```python
from build123d import *

# Parameters (mm, degrees)
EXTRUDE_1_DEPTH      = 7
SKETCH_4_W           = 12.5
SKETCH_4_H           = 12.5
CUT_EXTRUDE_1_DEPTH  = 5.5
SKETCH_5_R           = 2.6
SKETCH_5_R_2         = 6.5
CUT_EXTRUDE_2_DEPTH  = 64.474798149
SKETCH_6_R           = 1
CUT_EXTRUDE_3_DEPTH  = 64.474798149
EXTRUDE_2_DEPTH      = 7
SKETCH_9_W           = 12
SKETCH_9_H           = 12
CUT_EXTRUDE_5_DEPTH  = 5
SKETCH_10_R          = 2.75
CUT_EXTRUDE_6_DEPTH  = 16
SKETCH_11_W          = 6.086395164
SKETCH_11_H          = 5.94224859
CUT_EXTRUDE_7_DEPTH  = 10
SKETCH_13_W          = 6.086395164
SKETCH_13_H          = 2.190675797
CUT_EXTRUDE_8_DEPTH  = 10
SKETCH_14_R          = 1.5
CUT_EXTRUDE_9_DEPTH  = 10
FILLET_1_R           = 0.3
FILLET_2_R           = 0.3
SKETCH_15_R          = 5
SKETCH_15_R_2        = 8.5
CUT_EXTRUDE_10_DEPTH = 1


with BuildPart() as part:
    # Эскиз1 → Бобышка-Вытянуть1 (new body)
    with BuildSketch(Plane.XY):
        with BuildLine():
            Line((0, 0), (50, 0))
            ThreePointArc((50, 0), (59.9, -9.9), (50, -19.8))
            Line((50, -19.8), (0, -19.8))
            ThreePointArc((0, -19.8), (-9.9, -9.9), (0, 0))
        make_face()
    extrude(amount=EXTRUDE_1_DEPTH)

    # Эскиз4 → Вырез-Вытянуть1 (cut)
    with BuildSketch(Plane.XY.offset(7)):
        with Locations((13.25, -9.9)):
            Rectangle(SKETCH_4_W, SKETCH_4_H)
        with Locations((28.75, -9.9)):
            Rectangle(SKETCH_4_W, SKETCH_4_H)
    extrude(amount=-CUT_EXTRUDE_1_DEPTH, mode=Mode.SUBTRACT)

    # Эскиз5 → Вырез-Вытянуть2 (cut, through all)
    with BuildSketch(Plane.XY.offset(7)):
        with Locations((0, -9.9)):
            Circle(SKETCH_5_R)
        with Locations((50, -9.9)):
            Circle(SKETCH_5_R_2)
    extrude(amount=-CUT_EXTRUDE_2_DEPTH, mode=Mode.SUBTRACT)

    # Эскиз6 → Вырез-Вытянуть3 (cut, through all)
    with BuildSketch(Plane.XY.offset(7)):
        with Locations((10.5, -3.65)):
            Circle(SKETCH_6_R)
        with Locations((15.5, -3.65)):
            Circle(SKETCH_6_R)
        with Locations((26, -3.65)):
            Circle(SKETCH_6_R)
        with Locations((31, -3.65)):
            Circle(SKETCH_6_R)
        with Locations((10.5, -16.15)):
            Circle(SKETCH_6_R)
        with Locations((15.5, -16.15)):
            Circle(SKETCH_6_R)
        with Locations((26, -16.15)):
            Circle(SKETCH_6_R)
        with Locations((31, -16.15)):
            Circle(SKETCH_6_R)
    extrude(amount=-CUT_EXTRUDE_3_DEPTH, mode=Mode.SUBTRACT)

    # Эскиз8 → Бобышка-Вытянуть2 (add)
    with BuildSketch(Plane.XY.offset(7)):
        with BuildLine():
            Line((0, 2.1), (50, 2.1))
            ThreePointArc((50, 2.1), (62, -9.9), (50, -21.9))
            Line((50, -21.9), (0, -21.9))
            ThreePointArc((0, -21.9), (-12, -9.9), (0, 2.1))
        make_face()
        with BuildLine():
            Line((0, -0.209438441), (50, -0.209438441))
            ThreePointArc((50, -0.209438441), (59.690561559, -9.9), (50, -19.590561559))
            Line((50, -19.590561559), (0, -19.590561559))
            ThreePointArc((0, -19.590561559), (-9.690561559, -9.9), (0, -0.209438441))
        make_face(mode=Mode.SUBTRACT)
    extrude(amount=-EXTRUDE_2_DEPTH)

    # Эскиз9 → Вырез-Вытянуть5 (cut)
    with BuildSketch(Plane(origin=(0, 0, 0), x_dir=(-1, 0, 0), z_dir=(0, 0, -1))):
        with Locations((0, -9.9)):
            Rectangle(SKETCH_9_W, SKETCH_9_H)
    extrude(amount=-CUT_EXTRUDE_5_DEPTH, mode=Mode.SUBTRACT)

    # Эскиз10 → Вырез-Вытянуть6 (cut)
    with BuildSketch(Plane.XZ.offset(21.9)):
        with Locations((39, 4.7)):
            Circle(SKETCH_10_R)
    extrude(amount=-CUT_EXTRUDE_6_DEPTH, mode=Mode.SUBTRACT)

    # Эскиз11 → Вырез-Вытянуть7 (cut)
    with BuildSketch(Plane.XZ.offset(21.9)):
        with Locations((39, 4.7)):
            Rectangle(SKETCH_11_W, SKETCH_11_H)
    extrude(amount=-CUT_EXTRUDE_7_DEPTH, mode=Mode.SUBTRACT)

    # Эскиз13 → Вырез-Вытянуть8 (cut)
    with BuildSketch(Plane.XY.offset(1.728875705)):
        with Locations((39, -20.804662101)):
            Rectangle(SKETCH_13_W, SKETCH_13_H)
    extrude(amount=-CUT_EXTRUDE_8_DEPTH, mode=Mode.SUBTRACT)

    # Эскиз14 → Вырез-Вытянуть9 (cut)
    with BuildSketch(Plane.XY.offset(7)):
        with Locations((21, -1.9)):
            Circle(SKETCH_14_R)
        with Locations((21, -17.9)):
            Circle(SKETCH_14_R)
        with Locations((43, -1.9)):
            Circle(SKETCH_14_R)
        with Locations((-7, -9.9857634)):
            Circle(SKETCH_14_R)
        with Locations((43, -17.9)):
            Circle(SKETCH_14_R)
    extrude(amount=-CUT_EXTRUDE_9_DEPTH, mode=Mode.SUBTRACT)

    # Скругление1
    fillet_1_edges = [part.edges().sort_by_distance(p)[0] for p in [
        (-6, -8.867729411, 2.5),
        (-6, -11.103797388, 2.5),
    ]]
    fillet(fillet_1_edges, radius=FILLET_1_R)

    # Скругление2
    fillet_2_edges = [part.edges().sort_by_distance(p)[0] for p in [
        (42.043197582, -16.744781781, 4.364437853),
        (42.043197582, -19.055218219, 4.364437853),
    ]]
    fillet(fillet_2_edges, radius=FILLET_2_R)

    # Эскиз15 → Вырез-Вытянуть10 (cut)
    with BuildSketch(Plane.XY.offset(7)):
        with Locations((0, -9.9)):
            Circle(SKETCH_15_R)
        with Locations((50, -9.9)):
            Circle(SKETCH_15_R_2)
    extrude(amount=-CUT_EXTRUDE_10_DEPTH, mode=Mode.SUBTRACT)


solid = part.part
```
Read the model definition and answer for the solid it produces. Units are mm, in the model's axes. A direction names the side the tool comes from. Coordinates: 2 decimals unless noted, no trailing zeros. Order: outer loops, then holes, each group sorted by start corner. A loop starts at its lowest first (then second) coordinate and runs counter-clockwise, first axis right, second up. Notation, with made-up numbers: (83, 17.25) - (131, 17.25) arc R11 ccw to (131, 37.25) - close; hole circle Ø2 at (-5, -11). An arc over 180 degrees is marked (long way). Answer as a JSON object with one key per item and string values. Group by question number.
Item 1: Section A-A (x = 15.5) is taken. Give the vertices of the cut face in (y, z).
Item 2: Section B-B (x = 29) is taken. Give the vertices of the cut face in (y, z).
Item 3: Section D-D (z = 3) is taken. State how many separate pieces and enclosed holes the cut face has, plus the area to 3 significant figures.
Item 4: A tool of negligible diameter and unlimited length cuts with its end or side. For faces 3 (the face through (0, -3.9, 2)), 4 (the face through (24, -16.15, 4)), 5 (the face through (39, -19.709, 1)), from which of +Z, -Z, +X, -X, +Y, -Y can it reach the whole face along a straight path? Write none if from no direction.
Item 5: Consider probe 1 along X at (y, z) = (-9.75, 1); probe 2 along Y at (x, z) = (31, 3.25); probe 3 along X at (y, z) = (-2, 3.25). Determine where each line is inside the solid, lowest interval first. Write a range as from..to.
Item 6: The mould has two halves that part along Z. Classify faces 1 (the face through (2, -12, 6)), 2 (the face through (33, -16.15, 4)): +Z half, -Z half, draft (parallel to the pull), parting line (faces both ways), or undercut.
Item 7: Flat-ended cylindrical pins translate along their axes: P1, Ø3.5, axis at y = -13, z = 3, coming from the +X side; P2, Ø3, axis at y = -4, z = 1, coming from the +X side; P3, Ø0.9, axis at x = 40, z = 1, coming from the -Y side; P4, Ø1.8, axis at x = 15.5, y = -16.15, coming from the +Z side. Find the tip coordinate at first contact, or state that the pin passes through.
Item 8: Section C-C (x = 51) is taken. Give the vertices of the cut face in (y, z).
Results are:
{
 "1": {"outline": "(-21.9, 0) - (-17.15, 0) - (-17.15, 7) - (-21.9, 7) - close; (-15.15, 0) - (-4.65, 0) - (-4.65, 1.5) - (-15.15, 1.5) - close; (-2.65, 0) - (2.1, 0) - (2.1, 7) - (-2.65, 7) - close"},
 "2": {"outline": "(-21.9, 0) - (2.1, 0) - (2.1, 7) - (-3.65, 7) - (-3.65, 1.5) - (-16.15, 1.5) - (-16.15, 7) - (-21.9, 7) - close"},
 "3": {"separate pieces": "1", "enclosed holes": "7", "area": "930 mm^2"},
 "4": {"face 3": "-Z", "face 4": "+Z", "face 5": "+Z, -Z, -Y"},
 "5": {"probe 1": "x = -12..-8.48, 6..43.5, 56.5..62", "probe 2": "y = -21.9..-17.15, -2.65..2.1", "probe 3": "x = -9.03..19.5, 22.5..41.5, 44.5..59.03"},
 "6": {"face 1": "+Z half", "face 2": "draft"},
 "7": {"P1": "stops at x = 61.92", "P2": "stops at x = 61.16", "P3": "stops at y = -19.71", "P4": "passes through"},
 "8": {"outline": "(-21.86, 0) - (-16.32, 0) - (-16.32, 6) - (-18.34, 6) - (-18.34, 7) - (-21.86, 7) - close; (-3.48, 0) - (2.06, 0) - (2.06, 7) - (-1.46, 7) - (-1.46, 6) - (-3.48, 6) - close"}
}
